Here's how the part is built. I have some questions about the finished solid (model axes, mm). Face numbers are marked on the shaded views. A direction names the side the tool comes from. Coordinates: 2 decimals unless noted, no trailing zeros. Write each loop counter-clockwise with the first axis right and the second up, starting at its lowest first coordinate (ties: lowest second). Pieces come first, ordered by that corner, then holes.
Item 1: If I drill on line 1 (Z direction, x = -0.5, y = -5); line 2 (X direction, y = -2.5, z = 8.25); line 3 (Z direction, x = 4.75, y = -2.75), over which ranges is the centre line in solid material (lowest first)?
Item 2: If we section it at D-D (y = -3): Please give me the cut outline in (x, z).
Item 3: For the marked faces 4, 5 and 6, which set-ups out of +Z, -Z, +X, -X, +Y, -Y let a thin tool reach every point of the face, with its end or its side?
Item 4: If we section it at A-A (y = -8.7): Please give me the cut outline in (x, z).
Item 5: If we section it at B-B (z = 0.75): Please give me the cut outline in (x, y), then the cut area to 3 significant figures.
Item 6: We'd pull the mould along X, two halves only. Please class the marked faces 1, 2 and 3: +X half, -X half, draft (parallel to the pull), parting line (faces both ways), or undercut.
Item 7: I'm going to push flat-ended pins straight in: pin 1 Ø5.5 at (y, z) = (-5, 7.5) entering from +X; pin 2 Ø5 at (x, z) = (7.5, 5) entering from -Y; pin 3 Ø5 at (y, z) = (-2, 5.5) entering from -X; pin 4 Ø2 at (x, z) = (5.5, 0.5) entering from -Y. Where does each tip first touch, or does it pass through?
Item 8: If we section it at C-C (x = 3): Please give me the cut outline in (y, z).
from build123d import *

# Parameters (mm, degrees)
F0_W     = 5.9
F0_H     = 7
F0_W_2   = 8.4
F1_DEPTH = 1.8
F0_H_2   = 5.6
F2_DEPTH = 10.8
F3_SIZE  = 2
F4_R     = 1
F5_DEPTH = 0.8
F7_DEPTH = 2.601
F8_W     = 2
F8_H     = 1.7
F8_W_2   = 6.1
F9_DEPTH = 14.301
F10_R    = 2.6


# Not quite as in the source:
# - a pattern or mirror of a feature is missing from the dataset's text; its kind, count and spacing are read off the source's solid


with BuildPart() as f1:
    # F0 (on Top) → F1 (new body)
    with BuildSketch(Plane.XY):
        with Locations((-7.15, -3.5)):
            Rectangle(F0_W, F0_H)
        with Locations((0, -3.5)):
            Rectangle(F0_W_2, F0_H)
        with Locations((7.15, -3.5)):
            Rectangle(F0_W, F0_H)
    extrude(amount=F1_DEPTH)

    # F0 (on Top) → F2 (join)
    with BuildSketch(Plane.XY):
        with Locations((0, -9.8)):
            Rectangle(F0_W_2, F0_H_2)
        with Locations((0, -3.5)):
            Rectangle(F0_W_2, F0_H)
    extrude(amount=F2_DEPTH)

    # F3
    f3_edges = [f1.edges().sort_by_distance(p)[0] for p in [
        (-4.2, -12.6, 5.4),
        (4.2, -12.6, 5.4),
    ]]
    chamfer(f3_edges, length=F3_SIZE)

    # F4 (on face) → F5 (join)
    with BuildSketch(Plane(origin=(0, 0, 0), x_dir=(1, 0, 0), z_dir=(0, 0, -1))):
        with Locations((0, 2.3)):
            Circle(F4_R)
        with Locations((0, 8.7)):
            Circle(F4_R)
    extrude(amount=F5_DEPTH)

    # F6 (on face) → F7 (cut, through all)
    with BuildSketch(Plane.XY.offset(1.8)):
        with BuildLine():
            Line((8.9, -3.7), (8.9, -2.3))
            ThreePointArc((8.9, -2.3), (7.5, -0.9), (6.1, -2.3))
            Line((6.1, -2.3), (6.1, -3.7))
            ThreePointArc((6.1, -3.7), (7.5, -5.1), (8.9, -3.7))
        make_face()
    f7 = extrude(amount=-F7_DEPTH, mode=Mode.SUBTRACT)

    # F7_copies: F7 across plane
    add(f7.mirror(Plane(origin=(0, 0, 0), x_dir=(0, 0, -1), z_dir=(-1, 0, 0))), mode=Mode.SUBTRACT)

    # F8 (on face) → F9 (cut, through all)
    with BuildSketch(Plane(origin=(-4.2, 0, 0), x_dir=(0, -1, 0), z_dir=(-1, 0, 0))):
        with Locations((11.6, 4.75)):
            Rectangle(F8_W, F8_H)
        with Locations((7.55, 4.75)):
            Rectangle(F8_W_2, F8_H)
    extrude(amount=-F9_DEPTH, mode=Mode.SUBTRACT)

    # F10
    f10_edges = [f1.edges().sort_by_distance(p)[0] for p in [
        (-10.1, -7, 0.9),
        (-10.1, 0, 0.9),
        (10.1, -7, 0.9),
        (10.1, 0, 0.9),
    ]]
    fillet(f10_edges, radius=F10_R)


solid = f1.part
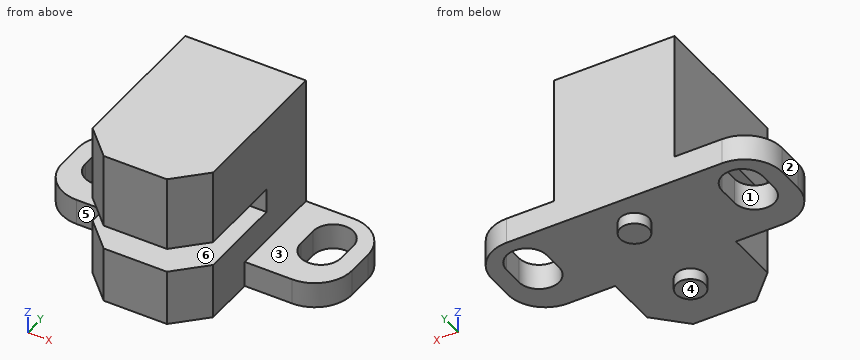
Answer list:
1. line 1: z = 0 to 3.9, 5.6 to 10.8
1. line 2: x = -4.2 to 4.2
1. line 3: z = 0 to 1.8
2. outline: (-10.1, 0) - (-8.9, 0) - (-8.9, 1.8) - (-10.1, 1.8) - close; (-6.1, 0) - (-0.71, 0) - (-0.71, -0.8) - (0.71, -0.8) - (0.71, 0) - (6.1, 0) - (6.1, 1.8) - (4.2, 1.8) - (4.2, 10.8) - (-4.2, 10.8) - (-4.2, 1.8) - (-6.1, 1.8) - close; (8.9, 0) - (10.1, 0) - (10.1, 1.8) - (8.9, 1.8) - close
3. face 4: -Z, +X, -X, +Y, -Y
3. face 5: +Z, -Z, -X, -Y
3. face 6: +X, -X, -Y
4. outline: (-4.2, 0) - (-1, 0) - (-1, -0.8) - (1, -0.8) - (1, 0) - (4.2, 0) - (4.2, 3.9) - (-4.2, 3.9) - close; (-4.2, 5.6) - (4.2, 5.6) - (4.2, 10.8) - (-4.2, 10.8) - close
5. outline: (-10.1, -4.4) arc R2.6 ccw to (-7.5, -7) - (-4.2, -7) - (-4.2, -10.6) - (-2.2, -12.6) - (2.2, -12.6) - (4.2, -10.6) - (4.2, -7) - (7.5, -7) arc R2.6 ccw to (10.1, -4.4) - (10.1, -2.6) arc R2.6 ccw to (7.5, 0) - (-7.5, 0) arc R2.6 ccw to (-10.1, -2.6) - close; hole (-8.9, -3.7) arc R1.4 ccw to (-6.1, -3.7) - (-6.1, -2.3) arc R1.4 ccw to (-8.9, -2.3) - close; hole (6.1, -3.7) arc R1.4 ccw to (8.9, -3.7) - (8.9, -2.3) arc R1.4 ccw to (6.1, -2.3) - close
5. area: 158 mm2
6. face 1: undercut
6. face 2: -X half
6. face 3: draft
7. pin 1: stops at x = 4.2
7. pin 2: passes through
7. pin 3: stops at x = -4.2
7. pin 4: stops at y = -7
8. outline: (-11.8, 0) - (0, 0) - (0, 10.8) - (-11.8, 10.8) - (-11.8, 5.6) - (-4.5, 5.6) - (-4.5, 3.9) - (-11.8, 3.9) - close
